Autodesk Inventor part; units mm, degrees
ref_plane "YZ Plane" through (0, 0, 0) normal (1, 0, 0) x (0, 1, 0)
ref_plane "XZ Plane" through (0, 0, 0) normal (0, 1, 0) x (-1, 0, 0)
ref_plane "XY Plane" through (0, 0, 0) normal (0, 0, 1) x (1, 0, 0)
sketch "Sketch1" plane through (0, 0, 0) normal (0, 1, 0) x (-1, 0, 0)
  line L0 (14.5, 7) -> (-14.5, 7)
  line L1 (-14.5, 7) -> (-14.5, -7)
  line L2 (-14.5, -7) -> (14.5, -7)
  line L3 (14.5, -7) -> (14.5, 7)
  point P0 (0, 0)
  dimension "d0" = 14
  dimension "d1" = 29
  dimension "d2" = 14.5
  dimension "d3" = 7
extrude "Extrusion1" add sketch "Sketch1" along normal blind 10
fillet "Fillet1" radius 1 4 edges at (14.5, 5, 7) (14.5, 5, -7) (-14.5, 5, -7) (-14.5, 5, 7)
shell "Shell1" thickness 1.5 removed faces 1 at (4.5, 0, 2.3333)
sketch "Sketch3" plane through (0, 10, 0) normal (0, 1, 0) x (1, 0, 0)
  line L0 (-10.5, -3) -> (-4.5, -3)
  line L1 (-4.5, -3) -> (-4.5, 3)
  line L2 (-4.5, 3) -> (-10.5, 3)
  line L3 (-10.5, 3) -> (-10.5, -3)
  line L4 (4.5, -3) -> (10.5, -3)
  line L5 (10.5, -3) -> (10.5, 3)
  line L6 (10.5, 3) -> (4.5, 3)
  line L7 (4.5, 3) -> (4.5, -3)
  line L8 (-13.5, -7) -> (13.5, -7)
  line L9 (-14.5, 6) -> (-14.5, -6)
  line L10 (14.5, -6) -> (14.5, 6)
  point P0 (0, 0)
  dimension "d14" = 6
  dimension "d15" = 6
  dimension "d16" = 4
  dimension "d17" = 4
  dimension "d18" = 4
  dimension "d19" = 6
extrude "Extrusion3" cut sketch "Sketch3" against normal through all
sketch "Sketch4" plane through (0, 0, 0) normal (0, -1, 0) x (1, 0, 0)
  line L0 (11.5, 6.75) -> (3.5, 6.75)
  line L1 (3.5, 6.75) -> (3.5, 5.75)
  line L2 (3.5, 5.75) -> (11.5, 5.75)
  line L3 (11.5, 5.75) -> (11.5, 6.75)
  line L4 (-3.5, 6.75) -> (-11.5, 6.75)
  line L5 (-11.5, 6.75) -> (-11.5, 5.75)
  line L6 (-11.5, 5.75) -> (-3.5, 5.75)
  line L7 (-3.5, 5.75) -> (-3.5, 6.75)
  line L8 (11.5, -5.75) -> (3.5, -5.75)
  line L9 (3.5, -5.75) -> (3.5, -6.75)
  line L10 (3.5, -6.75) -> (11.5, -6.75)
  line L11 (11.5, -6.75) -> (11.5, -5.75)
  line L12 (-3.5, -5.75) -> (-11.5, -5.75)
  line L13 (-11.5, -5.75) -> (-11.5, -6.75)
  line L14 (-11.5, -6.75) -> (-3.5, -6.75)
  line L15 (-3.5, -6.75) -> (-3.5, -5.75)
  line L16 (14.5, 6) -> (14.5, -6)
  line L17 (-14.5, -6) -> (-14.5, 6)
  line L18 (-13, 5.5) -> (13, 5.5)
  line L19 (13.5, -7) -> (-13.5, -7)
  point P0 (0, 0)
  dimension "d22" = 3
  dimension "d23" = 3
  dimension "d24" = 1
  dimension "d25" = 8
  dimension "d26" = 1
  dimension "d27" = 8
  dimension "d28" = 0.25
  dimension "d29" = 0.25
extrude "Extrusion4" add sketch "Sketch4" along normal blind 1.5
sketch "Sketch5" plane through (14.5, 0, 6) normal (1, 0, 0) x (0, 0, -1)
  line L0 (0, 0) -> (12, 0)
  line L1 (2, 2) -> (10, 2)
  line L2 (10, 2) -> (10, 0)
  line L3 (10, 0) -> (2, 0)
  line L4 (2, 0) -> (2, 2)
  line L5 (0, 0) -> (0, 10)
  point P0 (6, 0)
  point P1 (2, 0)
  dimension "d32" = 8
  dimension "d33" = 2
  dimension "d34" = 2
extrude "Extrusion5" cut sketch "Sketch5" against normal blind 1.5
properties part number "Keyboard_Base"
Can you work these out from the model? Positions are in its coordinate system, mm. A direction names the side the tool comes from. Coordinates: 2 decimals unless noted, no trailing zeros. Loops run counter-clockwise (first coordinate to the right, second up) from the corner with the lowest first, then second, coordinate; pieces in that order, holes last. Notation, with made-up numbers: (56, 67.5) - (86, 67.5) arc R21 ccw to (86, 104.5) - close; hole circle Ø3 at (78.25, 63). An arc over 180 degrees is marked (long way). Use a Markdown table: item, result.
Item 1: Will these pins go through, and if not, where does the flat tip stop? pin 1 (0.5 mm diameter, centred on y = -0.5, z = 6.5, fed in from -X); pin 2 (1.6 mm diameter, centred on x = 8, y = -1, fed in from -Z); pin 3 (0.8 mm diameter, centred on x = -8, y = -1, fed in from +Z).
Numbers:
| item | result |
|---|---|
| pin 1 | stops at x = -11.5 |
| pin 2 | stops at z = -6.75 |
| pin 3 | stops at z = 6.75 |
Item 2: We'd pull the mould along X, two halves only. Please class faces 1 (the face through (14, 2, 0)), 2 (the face through (-11.5, -1, -6)), 3 (the face through (-7, 9, -3)): released by +X, released by -X, zero draft, split by the parting line, or undercut.
Numbers:
| item | result |
|---|---|
| face 1 | zero draft |
| face 2 | released by -X |
| face 3 | undercut |
Item 3: I want a section at C-C on x = -8.75. Please give me the cut outline in (y, z), and give its area (3 significant figures).
Numbers:
| item | result |
|---|---|
| outline | (-1.5, -6.75) - (0, -6.75) - (0, -7) - (10, -7) - (10, -3) - (8.5, -3) - (8.5, -5.5) - (0, -5.5) - (0, -5.75) - (-1.5, -5.75) - close; (-1.5, 5.75) - (0, 5.75) - (0, 5.5) - (8.5, 5.5) - (8.5, 3) - (10, 3) - (10, 7) - (0, 7) - (0, 6.75) - (-1.5, 6.75) - close |
| area | 40.5 mm2 |
Item 4: I want a section at A-A on z = 2.5. Please give me the cut outline in (x, y), and give its area (3 significant figures).
Numbers:
| item | result |
|---|---|
| outline | (-14.5, 0) - (-13, 0) - (-13, 8.5) - (-10.5, 8.5) - (-10.5, 10) - (-14.5, 10) - close; (-4.5, 8.5) - (4.5, 8.5) - (4.5, 10) - (-4.5, 10) - close; (10.5, 8.5) - (13, 8.5) - (13, 2) - (14.5, 2) - (14.5, 10) - (10.5, 10) - close |
| area | 48.0 mm2 |
Item 5: I want a section at D-D on y = 9. Please give me the cut outline in (x, z), and give its area (3 significant figures).
Numbers:
| item | result |
|---|---|
| outline | (-14.5, -6) arc R1 ccw to (-13.5, -7) - (13.5, -7) arc R1 ccw to (14.5, -6) - (14.5, 6) arc R1 ccw to (13.5, 7) - (-13.5, 7) arc R1 ccw to (-14.5, 6) - close; hole (-10.5, -3) - (-4.5, -3) - (-4.5, 3) - (-10.5, 3) - close; hole (4.5, -3) - (10.5, -3) - (10.5, 3) - (4.5, 3) - close |
| area | 333 mm2 |
Item 6: If I drill on probe 1 along X at (y, z) = (3.5, 3.25); probe 2 along Z at (x, y) = (6, -0.5); probe 3 along Z at (x, y) = (1.25, 5), over which ranges is the centre line in solid material (lowest first)? Write a range as from..to.
Numbers:
| item | result |
|---|---|
| probe 1 | x = -14.5..-13, 13..14.5 |
| probe 2 | z = -6.75..-5.75, 5.75..6.75 |
| probe 3 | z = -7..-5.5, 5.5..7 |
Item 7: For faces 4 (the face through (0, 4, 5.5)), 5 (the face through (14, 1, -4)), 6 (the face through (7, -1, 5.75)), 7 (the face through (4.5, 9, 0)), 8 (the face through (-3.5, -1, 6)), which set-ups out of +Z, -Z, +X, -X, +Y, -Y let a thin tool reach every point of the face, with its end or its side?
Numbers:
| item | result |
|---|---|
| face 4 | -Y |
| face 5 | +X, -Y |
| face 6 | +X, -X, -Y |
| face 7 | +Y, -Y |
| face 8 | +Z, -Z, -Y |
Item 8: I want a section at B-B on y = 4.25. Please give me the cut outline in (x, z).
Numbers:
| item | result |
|---|---|
| outline | (-14.5, -6) arc R1 ccw to (-13.5, -7) - (13.5, -7) arc R1 ccw to (14.5, -6) - (14.5, 6) arc R1 ccw to (13.5, 7) - (-13.5, 7) arc R1 ccw to (-14.5, 6) - close; hole (-13, -5.5) - (13, -5.5) - (13, 5.5) - (-13, 5.5) - close |
